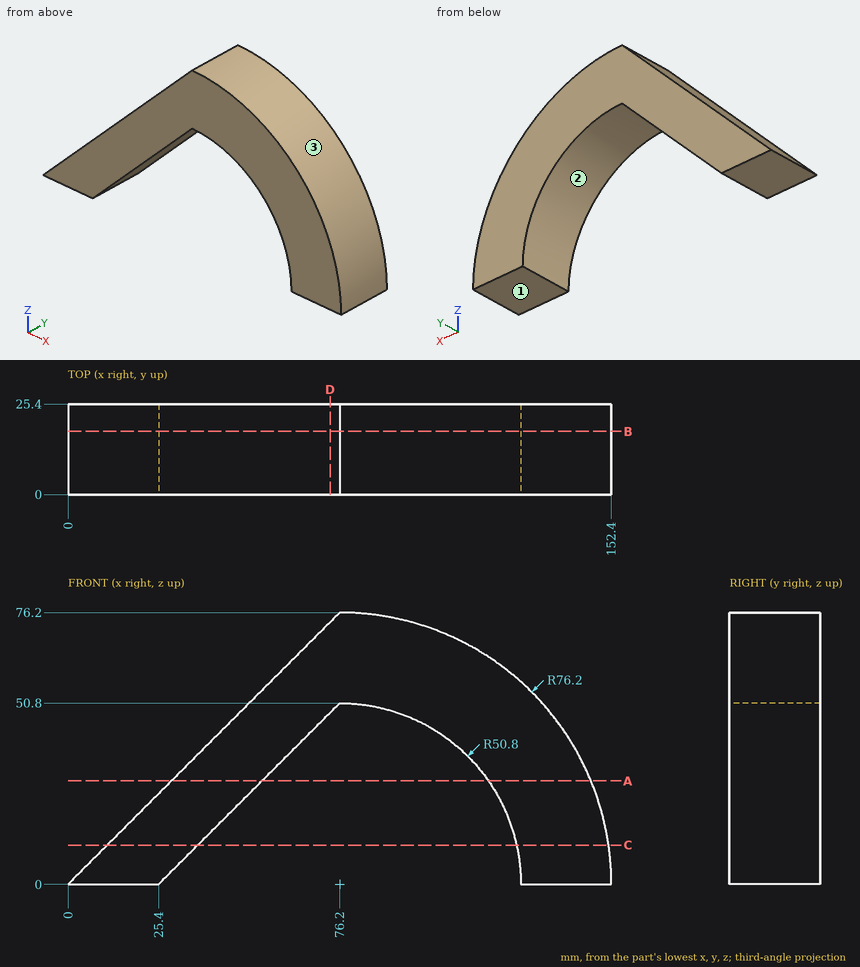
The drawing under review shows one solid part. Ordinate dimensions are in mm from its lowest x, y, z. Give positions to 0.01 mm unless a question says otherwise; leave off trailing zeros. Loops run counter-clockwise (first coordinate to the right, second up) from the corner with the lowest first, then second, coordinate; pieces in that order, holes last. Notation, with made-up numbers: M 59,42.5 L 66,42.5 A15 ccw 66,46.5 Z; hole C 32,7.25 d2. An arc over 180 degrees is marked long. Return JSON: item names as keys, results as strings. Group by question number.
Item 1: We need section B-B (y = 17.75). Give the boundary of the cut face in (x, z), and give its area (3 significant figures).
Item 2: We need section D-D (x = 73.5). Give the boundary of the cut face in (y, z).
Item 3: We need section C-C (z = 11). Give the boundary of the cut face in (x, y), and give its area (3 significant figures).
Item 4: Insertion check: pin 1 Ø1 at (y, z) = (19, 62.5) entering from -X; pin 2 Ø6 at (x, y) = (45, 17) entering from -Z; pin 3 Ø4 at (y, z) = (8.5, 8.5) entering from +X. Each pin has a flat end and moves straight along its axis. Give the tip position at first contact, or say it passes through.
Item 5: Mouldability with a two-part tool opening along X and no side actions: class the marked faces 1, 2 and 3 as released by +X, released by -X, zero draft, split by the parting line, or undercut.
Item 6: We need section A-A (z = 29). Give the boundary of the cut face in (x, y).
Item 7: For probe 1 along Z at (x, y) = (77.5, 10.5); probe 2 along X at (y, z) = (14.5, 16); probe 3 along X at (y, z) = (14.5, 40), list the stretches that pass through material, from the lowest coordinate up.
Output:
{
 "1": {"outline": "M 0,0 L 25.4,0 L 76.2,50.8 A50.8 cw 127,0 L 152.4,0 A76.2 ccw 76.2,76.2 Z", "area": "4,150 mm^2"},
 "2": {"outline": "M 0,48.1 L 25.4,48.1 L 25.4,73.5 L 0,73.5 Z"},
 "3": {"outline": "M 11,0 L 36.4,0 L 36.4,25.4 L 11,25.4 Z; M 125.79,0 L 151.6,0 L 151.6,25.4 L 125.79,25.4 Z", "area": "1,300 mm^2"},
 "4": {"pin 1": "stops at x = 62", "pin 2": "stops at z = 16.6", "pin 3": "stops at x = 152.12"},
 "5": {"face 1": "zero draft", "face 2": "undercut", "face 3": "released by +X"},
 "6": {"outline": "M 29,0 L 54.4,0 L 54.4,25.4 L 29,25.4 Z; M 117.91,0 L 146.67,0 L 146.67,25.4 L 117.91,25.4 Z"},
 "7": {"probe 1": "z = 50.78 to 76.19", "probe 2": "x = 16 to 41.4, 124.41 to 150.7", "probe 3": "x = 40 to 65.4, 107.52 to 141.06"}
}
